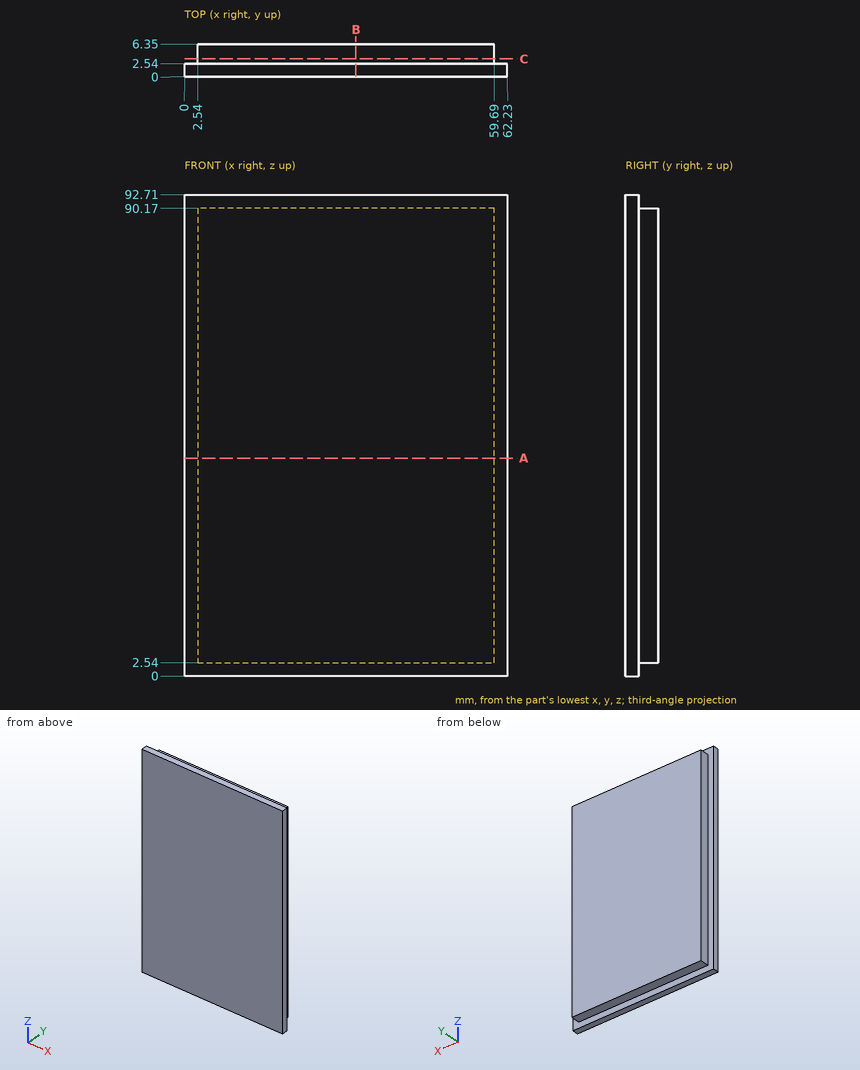
Design review of the part shown in the three views and the two pictorial views. Dimensions are in mm from the part's minimum x, y and z. Round coordinates to 2 decimals unless told otherwise and drop trailing zeros. Write each loop counter-clockwise with the first axis right and the second up, starting at its lowest first coordinate (ties: lowest second). Pieces come first, ordered by that corner, then holes.
Item 1: Consider section B-B on x = 33. Give the boundary of the cut face in (y, z), and give its area (3 significant figures).
Item 2: Consider section A-A on z = 42. Give the boundary of the cut face in (x, y), and give its area (3 significant figures).
Item 3: Consider section C-C on y = 3.5. Give the boundary of the cut face in (x, z), and give its area (3 significant figures).
Item 4: For pin 1 Ø10 at (x, z) = (20.5, 66.5) entering from -Y; pin 2 Ø1.9 at (x, y) = (18.5, 4) entering from +Z; pin 3 Ø1.1 at (x, y) = (34, 5) entering from -Z; pin 4 Ø1.1 at (y, z) = (4.5, 60) entering from +X, all flat-tipped, find the tip position at first contact; note any pin that passes through.
Item 5: Wall thickness on L1, parallel to Z at x = 6, y = 5.5; L2, parallel to X at y = 6.25, z = 56.5: over which ranges is each line inside the solid? List them lowest first.
Check values:
1. outline: (0, 0) - (2.54, 0) - (2.54, 2.54) - (6.35, 2.54) - (6.35, 90.17) - (2.54, 90.17) - (2.54, 92.71) - (0, 92.71) - close
1. area: 569 mm2
2. outline: (0, 0) - (62.23, 0) - (62.23, 2.54) - (59.69, 2.54) - (59.69, 6.35) - (2.54, 6.35) - (2.54, 2.54) - (0, 2.54) - close
2. area: 376 mm2
3. outline: (2.54, 2.54) - (59.69, 2.54) - (59.69, 90.17) - (2.54, 90.17) - close
3. area: 5,010 mm2
4. pin 1: stops at y = 0
4. pin 2: stops at z = 90.17
4. pin 3: stops at z = 2.54
4. pin 4: stops at x = 59.69
5. L1: z = 2.54 to 90.17
5. L2: x = 2.54 to 59.69
